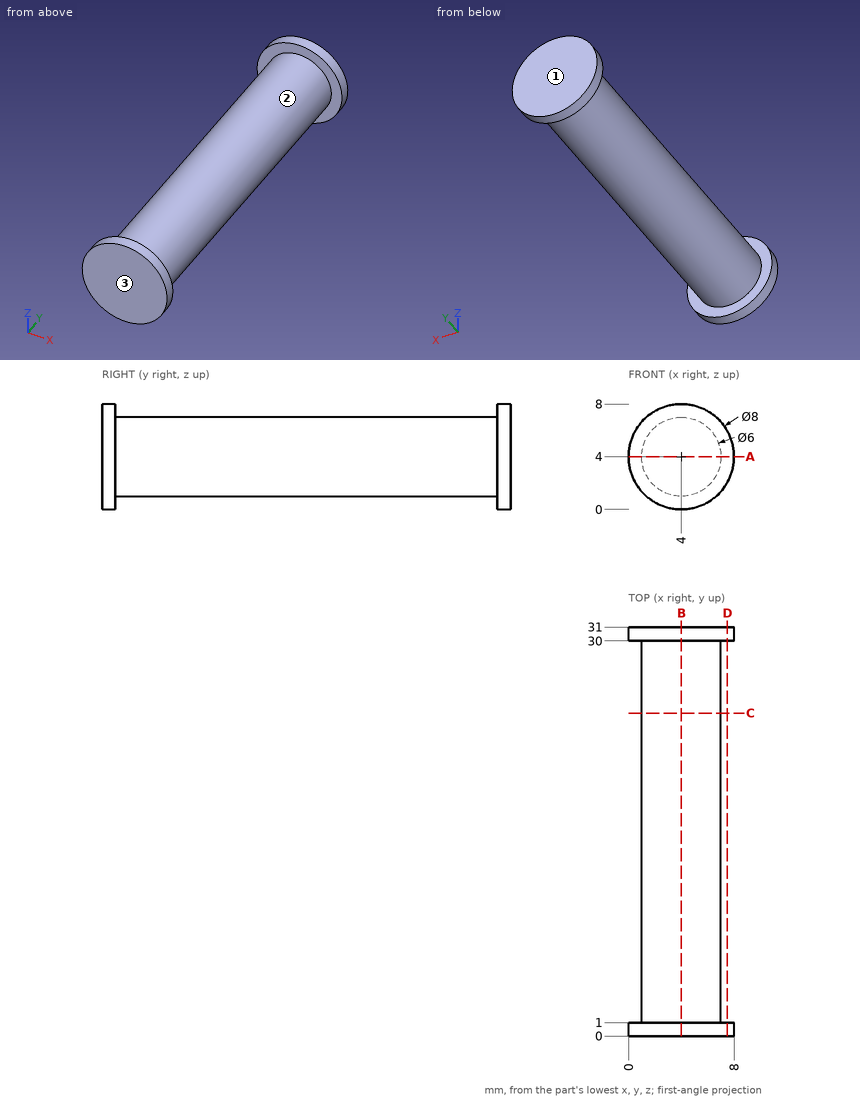
Job drawing, mm, ordinate dimensions from the low corner. One solid piece. Give positions to 0.01 mm unless a question says otherwise; leave off trailing zeros. Write each loop counter-clockwise with the first axis right and the second up, starting at its lowest first coordinate (ties: lowest second). Pieces come first, ordered by that corner, then holes. Notation, with made-up numbers: (74, 48.5) - (106, 48.5) arc R25 cw to (106, 82.5) - close; hole circle Ø7 at (79.5, 15). An arc over 180 degrees is marked (long way). Use one line per item in the form item = value. Start each with the question number.
1. Probe line 1 (Y direction, x = 4.25, z = 7.25); line 2 (X direction, y = 27.5, z = 4); line 3 (X direction, y = 26, z = 6). List the from-to ranges inside material, lowest first. Write a range as [from, to].
2. Band-saw the part on C-C on y = 24.5. Write the cut outline in (x, z), plus the area to 3 significant figures.
3. Drop flat-ended pins along their axis: pin 1 Ø4 at (x, y) = (6, 24.5) entering from -Z; pin 2 Ø1.5 at (y, z) = (16, 5) entering from -X; pin 3 Ø1.5 at (y, z) = (17, 5.5) entering from -X. Give the stop position or say it passes through.
4. Band-saw the part on A-A on z = 4. Write the cut outline in (x, y).
5. Band-saw the part on B-B on x = 4. Write the cut outline in (y, z), plus the area to 3 significant figures.
6. Band-saw the part on D-D on x = 7.5. Write the cut outline in (y, z), plus the area to 3 significant figures.
7. Two-plate mould, pull along Y, no slides. Class the marked faces 1, 2 and 3: released by +Y, released by -Y, zero draft, split by the parting line, or undercut.
Conclusion:
q1.line_1 = [0, 1], [30, 31]
q1.line_2 = [1, 7]
q1.line_3 = [1.76, 6.24]
q2.outline = circle Ø6 at (4, 4)
q2.area = 28.3 mm²
q3.pin_1 = 1
q3.pin_2 = 1.01
q3.pin_3 = 1.1
q4.outline = (0, 0) - (8, 0) - (8, 1) - (7, 1) - (7, 30) - (8, 30) - (8, 31) - (0, 31) - (0, 30) - (1, 30) - (1, 1) - (0, 1) - close
q5.outline = (0, 0) - (1, 0) - (1, 1) - (30, 1) - (30, 0) - (31, 0) - (31, 8) - (30, 8) - (30, 7) - (1, 7) - (1, 8) - (0, 8) - close
q5.area = 190 mm²
q6.outline = (0, 2.06) - (1, 2.06) - (1, 5.94) - (0, 5.94) - close; (30, 2.06) - (31, 2.06) - (31, 5.94) - (30, 5.94) - close
q6.area = 7.75 mm²
q7.face_1 = released by +Y
q7.face_2 = undercut
q7.face_3 = released by -Y
